```python
from build123d import *

# Parameters (mm, degrees)
SKETCH1_W           = 15
SKETCH1_H           = 15
BOSS_EXTRUDE2_DEPTH = 200
SKETCH2_W           = 15
SKETCH2_H           = 15
BOSS_EXTRUDE3_DEPTH = 215
SKETCH3_W           = 15
SKETCH3_H           = 15
BOSS_EXTRUDE4_DEPTH = 215
SKETCH4_R           = 5
CUT_EXTRUDE1_DEPTH  = 313.699936041
SKETCH5_R           = 5
CUT_EXTRUDE3_DEPTH  = 313.699936041


with BuildPart() as part:
    # Sketch1 → Boss-Extrude2 (new body)
    with BuildSketch(Plane.XY):
        with BuildLine():
            ThreePointArc((-7.5, 99.718353376), (0, 100), (7.5, 99.718353376))
            Line((7.5, 99.718353376), (7.5, 107.5))
            Line((7.5, 107.5), (-7.5, 107.5))
            Line((-7.5, 107.5), (-7.5, 99.718353376))
        make_face()
        with BuildLine():
            Line((7.5, 92.5), (7.5, 99.718353376))
            ThreePointArc((7.5, 99.718353376), (0, 100), (-7.5, 99.718353376))
            Line((-7.5, 99.718353376), (-7.5, 92.5))
            Line((-7.5, 92.5), (7.5, 92.5))
        make_face()
        with BuildLine():
            ThreePointArc((-99.718353376, 7.5), (-100, 0), (-99.718353376, -7.5))
            Line((-99.718353376, -7.5), (-92.5, -7.5))
            Line((-92.5, -7.5), (-92.5, 7.5))
            Line((-92.5, 7.5), (-99.718353376, 7.5))
        make_face()
        with BuildLine():
            Line((-107.5, -7.5), (-99.718353376, -7.5))
            ThreePointArc((-99.718353376, -7.5), (-100, 0), (-99.718353376, 7.5))
            Line((-99.718353376, 7.5), (-107.5, 7.5))
            Line((-107.5, 7.5), (-107.5, -7.5))
        make_face()
        with BuildLine():
            ThreePointArc((-7.5, -99.718353376), (0, -100), (7.5, -99.718353376))
            Line((7.5, -99.718353376), (7.5, -92.5))
            Line((7.5, -92.5), (-7.5, -92.5))
            Line((-7.5, -92.5), (-7.5, -99.718353376))
        make_face()
        with BuildLine():
            Line((7.5, -107.5), (7.5, -99.718353376))
            ThreePointArc((7.5, -99.718353376), (0, -100), (-7.5, -99.718353376))
            Line((-7.5, -99.718353376), (-7.5, -107.5))
            Line((-7.5, -107.5), (7.5, -107.5))
        make_face()
        with Locations((100, 0)):
            Rectangle(SKETCH1_W, SKETCH1_H)
    extrude(amount=BOSS_EXTRUDE2_DEPTH)

    # Sketch2 → Boss-Extrude3 (add)
    with BuildSketch(Plane.XZ.offset(107.5)):
        with Locations((0, 192.5)):
            Rectangle(SKETCH2_W, SKETCH2_H)
    extrude(amount=-BOSS_EXTRUDE3_DEPTH)

    # Sketch3 → Boss-Extrude4 (add)
    with BuildSketch(Plane(origin=(107.5, 0, 0), x_dir=(0, 0, -1), z_dir=(1, 0, 0))):
        with Locations((-192.5, 0)):
            Rectangle(SKETCH3_W, SKETCH3_H)
    extrude(amount=-BOSS_EXTRUDE4_DEPTH)

    # Sketch4 → Cut-Extrude1 (cut, through all)
    with BuildSketch(Plane(origin=(107.5, 0, 0), x_dir=(0, 0, -1), z_dir=(1, 0, 0))):
        with Locations(Location((-10, 0, 0), (0, 0, 90))):
            Circle(SKETCH4_R)
    extrude(amount=-CUT_EXTRUDE1_DEPTH, mode=Mode.SUBTRACT)

    # Sketch5 → Cut-Extrude3 (cut, through all)
    with BuildSketch(Plane.XZ.offset(107.5)):
        with Locations((0, 20)):
            Circle(SKETCH5_R)
    extrude(amount=-CUT_EXTRUDE3_DEPTH, mode=Mode.SUBTRACT)


solid = part.part
```
CAD build for the part. Positions are in the model's coordinates, mm. A direction names the side the tool comes from. Coordinates: 2 decimals unless noted, no trailing zeros. Order: outer loops, then holes, each group sorted by start corner. A loop starts at its lowest first (then second) coordinate and runs counter-clockwise, first axis right, second up.
(1) Pin check, flat tip, straight feed: pin 1 Ø6 at (x, z) = (0, 20) entering from +Y. Stop position of the tip, or through.
Solution:
pin 1: passes through
(2) Mould opens along Y. For faces 6 (the face through (100.105, -0.651, 14.957)), 7 (the face through (0, -107.5, 99)), 8 (the face through (0, -100, 0)), 9 (the face through (0, 0, 185)) say: released by +Y, released by -Y, zero draft, split by the parting line, or undercut.
Solution:
face 6: undercut
face 7: released by -Y
face 8: zero draft
face 9: undercut
(3) Saw through at D-D, the plane x = 0. Write the cut outline in (y, z), and give its area (4 significant figures).
Solution:
outline: (-107.5, 0) - (-92.5, 0) - (-92.5, 15) - (-107.5, 15) - close; (-107.5, 25) - (-92.5, 25) - (-92.5, 185) - (92.5, 185) - (92.5, 25) - (107.5, 25) - (107.5, 200) - (-107.5, 200) - close; (92.5, 0) - (107.5, 0) - (107.5, 15) - (92.5, 15) - close
area: 8,475 mm2
(4) Saw through at A-A, the plane z = 10. Write the cut outline in (x, y).
Solution:
outline: (-107.5, -7.5) - (-92.5, -7.5) - (-92.5, -5) - (-107.5, -5) - close; (-107.5, 5) - (-92.5, 5) - (-92.5, 7.5) - (-107.5, 7.5) - close; (-7.5, -107.5) - (7.5, -107.5) - (7.5, -92.5) - (-7.5, -92.5) - close; (-7.5, 92.5) - (7.5, 92.5) - (7.5, 107.5) - (-7.5, 107.5) - close; (92.5, -7.5) - (107.5, -7.5) - (107.5, -5) - (92.5, -5) - close; (92.5, 5) - (107.5, 5) - (107.5, 7.5) - (92.5, 7.5) - close
(5) Which spindle directions (+Z, -Z, +X, -X, +Y, -Y) get a long thin tool onto all of the face, cutting with end or side? Do faces 1 (the face through (92.5, 0, 91)), 2 (the face through (-94, 7.5, 130)), 3 (the face through (7.5, -95, 122)), 4 (the face through (-94, -7.5, 130)), 5 (the face through (7.5, 94, 129)). Say none if no direction does.
Solution:
face 1: -Z, +Y, -Y
face 2: +Z, -Z, -X, +Y
face 3: +Z, -Z, +X, -Y
face 4: +Z, -Z, -X, -Y
face 5: +Z, -Z, +X, +Y
(6) Drill centre lines: L1, parallel to Z at x = 97, y = 0; L2, parallel to Z at x = 0, y = -101; L3, parallel to Y at x = -51.5, z = 190.5. Where is each one in solid material? Low to high.
Solution:
L1: z = 0 to 5, 15 to 200
L2: z = 0 to 15, 25 to 200
L3: y = -7.5 to 7.5
(7) Saw through at B-B, the plane y = 0. Write the cut outline in (x, z).
Solution:
outline: (-107.5, 0) - (-92.5, 0) - (-92.5, 5) - (-107.5, 5) - close; (-107.5, 15) - (-92.5, 15) - (-92.5, 185) - (92.5, 185) - (92.5, 15) - (107.5, 15) - (107.5, 200) - (-107.5, 200) - close; (92.5, 0) - (107.5, 0) - (107.5, 5) - (92.5, 5) - close
(8) Saw through at C-C, the plane z = 120. Write the cut outline in (x, y), and give its area (3 significant figures).
Solution:
outline: (-107.5, -7.5) - (-92.5, -7.5) - (-92.5, 7.5) - (-107.5, 7.5) - close; (-7.5, -107.5) - (7.5, -107.5) - (7.5, -92.5) - (-7.5, -92.5) - close; (-7.5, 92.5) - (7.5, 92.5) - (7.5, 107.5) - (-7.5, 107.5) - close; (92.5, -7.5) - (107.5, -7.5) - (107.5, 7.5) - (92.5, 7.5) - close
area: 900 mm2
